Drawing for the job (mm, zero at the part's lowest x, y, z). Round coordinates to 2 decimals unless told otherwise and drop trailing zeros. Write each loop counter-clockwise with the first axis right and the second up, starting at its lowest first coordinate (ties: lowest second). Pieces come first, ordered by that corner, then holes. Notation, with made-up numbers: (14.5, -15) -> (44.5, -15) arc R19 ccw to (44.5, -8) -> close; hole circle Ø1 at (59, -6.75). An arc over 180 degrees is marked (long way). One line per question, with ' | ' between items.
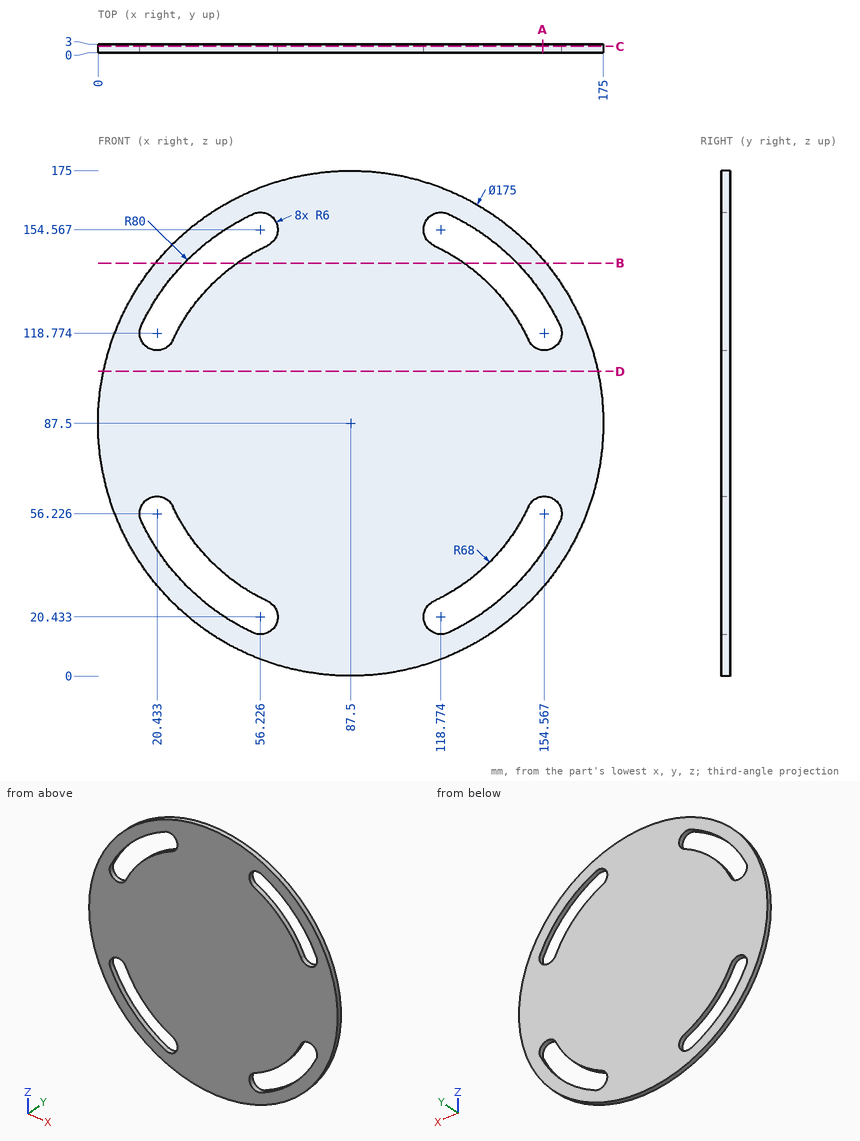
(1) Slice it at B-B (z = 143). Write the cut outline in (x, y).
Calculated:
outline: (19.85, 0) -> (29.88, 0) -> (29.88, 3) -> (19.85, 3) -> close; (48.21, 0) -> (126.79, 0) -> (126.79, 3) -> (48.21, 3) -> close; (145.12, 0) -> (155.15, 0) -> (155.15, 3) -> (145.12, 3) -> close
(2) Slice it at D-D (z = 105.5). Write the cut outline in (x, y).
Calculated:
outline: (1.87, 0) -> (173.13, 0) -> (173.13, 3) -> (1.87, 3) -> close
(3) Drop a flat-ended pin along its axis: pin 1 (1.5 mm diameter, centred on y = 2, z = 39.5, fed in from +X). Give the stop position or say it passes through.
Calculated:
pin 1: x = 161.15
(4) Wall check: line 1 (Z direction, x = 154, y = 0.95); line 2 (Z direction, x = 41, y = 1.05) (1 decimal); line 3 (X direction, y = 2.05, z = 124.5). Give the ranges that are in metal, low to high. Write a range as from..to.
Calculated:
line 1: 30.63..43.03, 62.2..112.8, 131.97..144.37 | line 2: 13.4..22.4, 37.9..137.1, 152.6..161.6 | line 3: 8.21..16.57, 30.45..144.55, 158.43..166.79
(5) Slice it at A-A (x = 154). Write the cut outline in (y, z).
Calculated:
outline: (0, 30.63) -> (3, 30.63) -> (3, 43.03) -> (0, 43.03) -> close; (0, 62.2) -> (3, 62.2) -> (3, 112.8) -> (0, 112.8) -> close; (0, 131.97) -> (3, 131.97) -> (3, 144.37) -> (0, 144.37) -> close
(6) Slice it at C-C (y = 2.15). Write the cut outline in (x, z) (1 decimal).
Calculated:
outline: circle Ø175 at (87.5, 87.5); hole (15, 53.7) arc R80 ccw to (53.7, 15) arc R6 ccw to (58.8, 25.9) arc R68 cw to (25.9, 58.8) arc R6 ccw to start; hole (15, 121.3) arc R6 ccw to (25.9, 116.2) arc R68 cw to (58.8, 149.1) arc R6 ccw to (53.7, 160) arc R80 ccw to start; hole (116.2, 25.9) arc R6 ccw to (121.3, 15) arc R80 ccw to (160, 53.7) arc R6 ccw to (149.1, 58.8) arc R68 cw to start; hole (116.2, 149.1) arc R68 cw to (149.1, 116.2) arc R6 ccw to (160, 121.3) arc R80 ccw to (121.3, 160) arc R6 ccw to start
